from build123d import *

# Parameters (mm, degrees)
SKETCH1_R                = 1
SKETCH1_R_2              = 2
SKETCH1_R_3              = 1.35
MAIN_PLATE_DEPTH         = 2
SKETCH2_R                = 2.5
SCREW_HOLES_DEPTH        = 1.7
SCREW_HOLES_CHAMFER_SIZE = 1.2


with BuildPart() as part:
    # Sketch1 → Main_plate (new body)
    with BuildSketch(Plane(origin=(0, 0, 0), x_dir=(1, 0, 0), z_dir=(0, 1, 0))):
        with BuildLine():
            Line((-85.7928409, -82.301697444), (-55.755812757, -142.75024532))
            ThreePointArc((-55.755812757, -142.75024532), (-54.140343173, -144.158373046), (-52.002337011, -144.011760212))
            ThreePointArc((-52.002337011, -144.011760212), (-3.951682628, -127.514559525), (46.728283967, -123.969985789))
            Line((46.728283967, -123.969985789), (137.274321343, -129.465618584))
            ThreePointArc((137.274321343, -129.465618584), (139.300267663, -128.766971907), (140.238810242, -126.840393723))
            Line((140.238810242, -126.840393723), (146.327388064, -26.524995005))
            ThreePointArc((146.327388064, -26.524995005), (145.628741387, -24.499048684), (143.702163203, -23.560506106))
            ThreePointArc((143.702163203, -23.560506106), (94.476527457, -18.20079206), (45.987943487, -8.163512858))
            ThreePointArc((45.987943487, -8.163512858), (45.725737799, -8.109235511), (45.459546448, -8.080252452))
            Line((45.459546448, -8.080252452), (27.492609364, -6.989760902))
            ThreePointArc((27.492609364, -6.989760902), (26.515953382, -7.103440368), (25.638814565, -7.547745919))
            ThreePointArc((25.638814565, -7.547745919), (8.167641381, -16.397587105), (-11.285751241, -18.661896472))
            ThreePointArc((-11.285751241, -18.661896472), (-12.626973233, -18.913649552), (-13.689904343, -19.76947284))
            ThreePointArc((-13.689904343, -19.76947284), (-45.694454746, -53.276077835), (-84.531326007, -78.548221698))
            ThreePointArc((-84.531326007, -78.548221698), (-85.939453733, -80.163691282), (-85.7928409, -82.301697444))
        make_face()
        with Locations(Location((24.759473712, -109.793011675, 0), (0, 0, 270))):
            Circle(SKETCH1_R, mode=Mode.SUBTRACT)
        with Locations(Location((35.739268597, -110.459423178, 0), (0, 0, 270))):
            Circle(SKETCH1_R, mode=Mode.SUBTRACT)
        with Locations(Location((45.493229955, -106.563189377, 0), (0, 0, 270))):
            Circle(SKETCH1_R_2, mode=Mode.SUBTRACT)
        with Locations(Location((143.003172699, -26.823913699, 0), (0, 0, 270))):
            Circle(SKETCH1_R_3, mode=Mode.SUBTRACT)
        with Locations(Location((73.916954773, -17.899251104, 0), (0, 0, 270))):
            Circle(SKETCH1_R_3, mode=Mode.SUBTRACT)
        with Locations(Location((-11.217743895, -21.971485999, 0), (0, 0, 270))):
            Circle(SKETCH1_R_3, mode=Mode.SUBTRACT)
        with Locations(Location((-82.615354782, -81.280438678, 0), (0, 0, 270))):
            Circle(SKETCH1_R_3, mode=Mode.SUBTRACT)
        with Locations(Location((-53.022766816, -140.834565069, 0), (0, 0, 270))):
            Circle(SKETCH1_R_3, mode=Mode.SUBTRACT)
        with Locations(Location((136.975163208, -126.141388687, 0), (0, 0, 270))):
            Circle(SKETCH1_R_3, mode=Mode.SUBTRACT)
        Polygon((47.520707964, -113.598943276), (52.411707503, -113.895799309), (52.145142902, -118.287717263), (47.254143363, -117.99086123), align=None, mode=Mode.SUBTRACT)
    extrude(amount=MAIN_PLATE_DEPTH)

    # Sketch2 → Screw_holes (cut)
    with BuildSketch(Plane.XZ):
        with Locations(Location((136.975163208, 126.141388687, 0), (0, 0, 270))):
            Circle(SKETCH2_R)
        with Locations(Location((-53.022766816, 140.834565069, 0), (0, 0, 270))):
            Circle(SKETCH2_R)
        with Locations(Location((-82.615354782, 81.280438678, 0), (0, 0, 270))):
            Circle(SKETCH2_R)
        with Locations(Location((-11.217743895, 21.971485999, 0), (0, 0, 270))):
            Circle(SKETCH2_R)
        with Locations(Location((73.916954773, 17.899251104, 0), (0, 0, 270))):
            Circle(SKETCH2_R)
        with Locations(Location((143.003172699, 26.823913699, 0), (0, 0, 270))):
            Circle(SKETCH2_R)
    extrude(amount=-SCREW_HOLES_DEPTH, mode=Mode.SUBTRACT)

    # Screw_holes_chamfer
    # the kernel refuses this chamfer: 1.2 mm, written as the material it adds along each edge
    with BuildSketch(Plane(origin=(143.003172699, 1.7, 26.823913699), x_dir=(0, 0, -1), z_dir=(-1, 0, 0))) as screw_holes_chamfer_piece_1_section:
        Polygon((2.5, SCREW_HOLES_CHAMFER_SIZE), (2.5 - SCREW_HOLES_CHAMFER_SIZE, 0), (2.5, 0), align=None)
    screw_holes_chamfer_piece_1 = revolve(axis=Axis((143.003172699, 1.7, 26.823913699), (0, -1, 0)), mode=Mode.PRIVATE)
    screw_holes_chamfer_piece_1 = screw_holes_chamfer_piece_1 - Plane(origin=(143.003172699, 1.073479929, 26.823913699), x_dir=(0, 0, 1), z_dir=(0, -1, 0)) * Cylinder(1.35, 10, mode=Mode.PRIVATE)
    add(screw_holes_chamfer_piece_1)
    with BuildSketch(Plane(origin=(73.916954773, 1.7, 17.899251104), x_dir=(0, 0, -1), z_dir=(-1, 0, 0))) as screw_holes_chamfer_piece_2_section:
        Polygon((2.5, SCREW_HOLES_CHAMFER_SIZE), (2.5 - SCREW_HOLES_CHAMFER_SIZE, 0), (2.5, 0), align=None)
    screw_holes_chamfer_piece_2 = revolve(axis=Axis((73.916954773, 1.7, 17.899251104), (0, -1, 0)), mode=Mode.PRIVATE)
    screw_holes_chamfer_piece_2 = screw_holes_chamfer_piece_2 - Plane(origin=(73.916954773, 1.073479929, 17.899251104), x_dir=(0, 0, 1), z_dir=(0, -1, 0)) * Cylinder(1.35, 10, mode=Mode.PRIVATE)
    add(screw_holes_chamfer_piece_2)
    with BuildSketch(Plane(origin=(-11.217743895, 1.7, 21.971485999), x_dir=(0, 0, -1), z_dir=(-1, 0, 0))) as screw_holes_chamfer_piece_3_section:
        Polygon((2.5, SCREW_HOLES_CHAMFER_SIZE), (2.5 - SCREW_HOLES_CHAMFER_SIZE, 0), (2.5, 0), align=None)
    screw_holes_chamfer_piece_3 = revolve(axis=Axis((-11.217743895, 1.7, 21.971485999), (0, -1, 0)), mode=Mode.PRIVATE)
    screw_holes_chamfer_piece_3 = screw_holes_chamfer_piece_3 - Plane(origin=(-11.217743895, 1.073479929, 21.971485999), x_dir=(0, 0, 1), z_dir=(0, -1, 0)) * Cylinder(1.35, 10, mode=Mode.PRIVATE)
    add(screw_holes_chamfer_piece_3)
    with BuildSketch(Plane(origin=(-82.615354782, 1.7, 81.280438678), x_dir=(0, 0, -1), z_dir=(-1, 0, 0))) as screw_holes_chamfer_piece_4_section:
        Polygon((2.5, SCREW_HOLES_CHAMFER_SIZE), (2.5 - SCREW_HOLES_CHAMFER_SIZE, 0), (2.5, 0), align=None)
    screw_holes_chamfer_piece_4 = revolve(axis=Axis((-82.615354782, 1.7, 81.280438678), (0, -1, 0)), mode=Mode.PRIVATE)
    screw_holes_chamfer_piece_4 = screw_holes_chamfer_piece_4 - Plane(origin=(-82.615354782, 1.073479929, 81.280438678), x_dir=(0, 0, 1), z_dir=(0, -1, 0)) * Cylinder(1.35, 11, mode=Mode.PRIVATE)
    add(screw_holes_chamfer_piece_4)
    with BuildSketch(Plane(origin=(-53.022766816, 1.7, 140.834565069), x_dir=(0, 0, -1), z_dir=(-1, 0, 0))) as screw_holes_chamfer_piece_5_section:
        Polygon((2.5, SCREW_HOLES_CHAMFER_SIZE), (2.5 - SCREW_HOLES_CHAMFER_SIZE, 0), (2.5, 0), align=None)
    screw_holes_chamfer_piece_5 = revolve(axis=Axis((-53.022766816, 1.7, 140.834565069), (0, -1, 0)), mode=Mode.PRIVATE)
    screw_holes_chamfer_piece_5 = screw_holes_chamfer_piece_5 - Plane(origin=(-53.022766816, 1.073479929, 140.834565069), x_dir=(0, 0, 1), z_dir=(0, -1, 0)) * Cylinder(1.35, 10, mode=Mode.PRIVATE)
    add(screw_holes_chamfer_piece_5)
    with BuildSketch(Plane(origin=(136.975163208, 1.7, 126.141388687), x_dir=(0, 0, -1), z_dir=(-1, 0, 0))) as screw_holes_chamfer_piece_6_section:
        Polygon((2.5, SCREW_HOLES_CHAMFER_SIZE), (2.5 - SCREW_HOLES_CHAMFER_SIZE, 0), (2.5, 0), align=None)
    screw_holes_chamfer_piece_6 = revolve(axis=Axis((136.975163208, 1.7, 126.141388687), (0, -1, 0)), mode=Mode.PRIVATE)
    screw_holes_chamfer_piece_6 = screw_holes_chamfer_piece_6 - Plane(origin=(136.975163208, 1.073479929, 126.141388687), x_dir=(0, 0, 1), z_dir=(0, -1, 0)) * Cylinder(1.35, 10, mode=Mode.PRIVATE)
    add(screw_holes_chamfer_piece_6)

    # Sketch4 → Cut-Loft1 section 0
    with BuildSketch(Plane(origin=(-7.640186202, 0, 125.879695971), x_dir=(0.9981631713309721, 0, 0.060582863901407005), z_dir=(-0.060582863901407005, 0, 0.9981631713309721))):
        with BuildLine():
            Line((34.465569885, 10.749979768), (39.265569885, 10.749979768))
            ThreePointArc((39.265569885, 10.749979768), (44.515569885, 5.499979768), (39.265569885, 0.249979768))
            Line((39.265569885, 0.249979768), (34.465569885, 0.249979768))
            ThreePointArc((34.465569885, 0.249979768), (29.215569885, 5.499979768), (34.465569885, 10.749979768))
        make_face()
    # Sketch3 → Cut-Loft1 section 1
    with BuildSketch(Plane(origin=(-7.337271882, 0, 120.888880114), x_dir=(0.9981631713309721, 0, 0.060582863901407005), z_dir=(-0.060582863901407005, 0, 0.9981631713309721))):
        with BuildLine():
            Line((34.465569885, 9.25), (39.265569885, 9.25))
            ThreePointArc((39.265569885, 9.25), (43.015590117, 5.499979768), (39.265569885, 1.749959536))
            Line((39.265569885, 1.749959536), (34.465569885, 1.749959536))
            ThreePointArc((34.465569885, 1.749959536), (30.715549653, 5.499979768), (34.465569885, 9.25))
        make_face()
    loft(mode=Mode.SUBTRACT)


solid = part.part
Could you check a few things on this model? Use its own coordinates, in mm. A direction names the side the tool comes from. Coordinates: 2 decimals unless noted, no trailing zeros. Order: outer loops, then holes, each group sorted by start corner. A loop starts at its lowest first (then second) coordinate and runs counter-clockwise, first axis right, second up. Notation, with made-up numbers: (-20, -28.5) -> (-5, -28.5) arc R12 cw to (-5, -8.5) -> close; hole circle Ø3 at (-4, 4). An arc over 180 degrees is marked (long way). One line per question, with ' | ' between items.
Q1. Imagine slicing it at A-A on y = 0.95. State how many separate pieces and enclosed holes the cut face has, and give its area (3 significant figures).
Return value:
separate pieces: 1 | enclosed holes: 10 | area: 22,500 mm²
Q2. I'm going to push flat-ended pins straight in: P1, Ø2, axis at x = 136.98, z = 126.14, coming from the -Y side; P2, Ø1, axis at y = 0.5, z = 46.5, coming from the -X side; P3, Ø4.5, axis at x = 143, z = 26.82, coming from the -Y side; P4, Ø1, axis at y = 1, z = 91, coming from the -X side. Where does each tip first touch, or does it pass through?
Return value:
P1: through | P2: x = -38.49 | P3: y = 0.74 | P4: x = -81.72
Q3. On a 3-axis mill with a long thin cutter (end or side, diameter ignored), from which of +Z, -Z, +X, -X, +Y, -Y can I reach the whole of each face in a straight line? I mean faces 4 (the face through (-13.436, 0.246, 20.818)), 5 (the face through (91.37, 0.99, 126.68)), 6 (the face through (143.24, 0.99, 77.38)). Say none if no direction works.
Return value:
face 4: -Y | face 5: +Z, +Y, -Y | face 6: +Z, +X, +Y, -Y
Q4. Imagine slicing it at C-C on x = -19. Please give me the cut outline in (y, z), and give its area (3 significant figures).
Return value:
outline: (0, 26.5) -> (2, 26.5) -> (2, 131.2) -> (0, 131.2) -> close | area: 209 mm²
Q5. Imagine slicing it at B-B on z = 37. Please give me the cut outline in (x, y), and give its area (3 significant figures).
Return value:
outline: (-28.29, 0) -> (145.69, 0) -> (145.69, 2) -> (-28.29, 2) -> close | area: 348 mm²
Q6. If I drill on L1, parallel to Z at x = -13.5, y = 0.4; L2, parallel to X at y = 0.1, z = 58.5; L3, parallel to Z at x = -29.5, y = 1.15, over which ranges is the centre line in solid material (lowest first)?
Return value:
L1: 19.54 to 20.95, 22.99 to 129.7 | L2: -52.27 to 144.39 | L3: 38.26 to 134.53
Q7. Thinking about a two-plate mould opening in X: for faces 1 (the face through (28, 2, 75)), 2 (the face through (95.16, 0.99, 18.31)), 3 (the face through (-4.65, 0.986, 127.658)), which applies, pulls with the +X half, pulls with the -X half, needs draft (parallel to the pull), parting line crosses it, or undercut?
Return value:
face 1: needs draft | face 2: pulls with the +X half | face 3: undercut
